```python
from build123d import *

# Parameters (mm, degrees)
SKETCH1_W           = 65
SKETCH1_H           = 100.5
BOSS_EXTRUDE1_DEPTH = 1.9
SKETCH2_W           = 35
SKETCH2_H           = 3
BOSS_EXTRUDE2_DEPTH = 2
FILLET2_R           = 1


with BuildPart() as part:
    # Sketch1 → Boss-Extrude1 (new body)
    with BuildSketch(Plane.XY):
        with Locations((34, 51.75)):
            Rectangle(SKETCH1_W, SKETCH1_H)
    extrude(amount=BOSS_EXTRUDE1_DEPTH)

    # Sketch2 → Boss-Extrude2 (add)
    with BuildSketch(Plane(origin=(0, 0, 0), x_dir=(-1, 0, 0), z_dir=(0, 0, -1))):
        with Locations((-34, 99)):
            Rectangle(SKETCH2_W, SKETCH2_H)
    extrude(amount=BOSS_EXTRUDE2_DEPTH)

    # Fillet2
    fillet2_edges = [part.edges().sort_by_distance(p)[0] for p in [
        (51.5, 99, 0),
        (34, 97.5, 0),
        (51.5, 97.5, -1),
        (16.5, 99, 0),
        (16.5, 97.5, -1),
        (51.5, 99, -2),
        (34, 97.5, -2),
        (16.5, 99, -2),
    ]]
    fillet(fillet2_edges, radius=FILLET2_R - 0.0001)  # a hair under: the kernel refuses the full size


solid = part.part
```
Check sheet for the modelled part. Datum: model origin and axes. Units: mm. A direction names the side the tool comes from. Round coordinates to 2 decimals unless told otherwise and drop trailing zeros. Loops run counter-clockwise (first coordinate to the right, second up) from the corner with the lowest first, then second, coordinate; pieces in that order, holes last. Notation, with made-up numbers: (-32.5, -10) -> (-12.5, -10) arc R30 cw to (-12.5, 14) -> close; hole circle Ø5 at (47, -27). An arc over 180 degrees is marked (long way). Answer in a Markdown table with one row per item.
Q1. Go/stop test with a flat-tipped pin: P1, Ø2, axis at x = 27, z = -1.5, coming from the +Y side. Record where the tip stops, or that it passes through.
Data:
| item | result |
|---|---|
| P1 | stops at y = 100.5 |
Q2. Thickness scan on L1, parallel to Z at x = 58.5, y = 37; L2, parallel to Y at x = 44, z = -0.3; L3, parallel to Y at x = 39.5, z = -0.5. Record the ranges inside material, lowest first.
Data:
| item | result |
|---|---|
| L1 | z = 0 to 1.9 |
| L2 | y = 97.21 to 100.5 |
| L3 | y = 97.37 to 100.5 |
Q3. Sectioned sample at C-C on x = 14. Enter the section's corners in (y, z), then the cut area to 3 significant figures.
Data:
| item | result |
|---|---|
| outline | (1.5, 0) -> (102, 0) -> (102, 1.9) -> (1.5, 1.9) -> close |
| area | 191 mm^2 |
Q4. Set-up check for faces 1 (the face through (1.5, 51, 1)), 2 (the face through (34, 100.5, -1)): record each of +Z, -Z, +X, -X, +Y, -Y from which the full face is reachable in a straight line by a thin tool's end or side.
Data:
| item | result |
|---|---|
| face 1 | +Z, -Z, -X, +Y, -Y |
| face 2 | -Z, +X, -X, +Y |
Q5. Sectioned sample at B-B on y = 47. Enter the section's corners in (x, z).
Data:
| item | result |
|---|---|
| outline | (1.5, 0) -> (66.5, 0) -> (66.5, 1.9) -> (1.5, 1.9) -> close |
